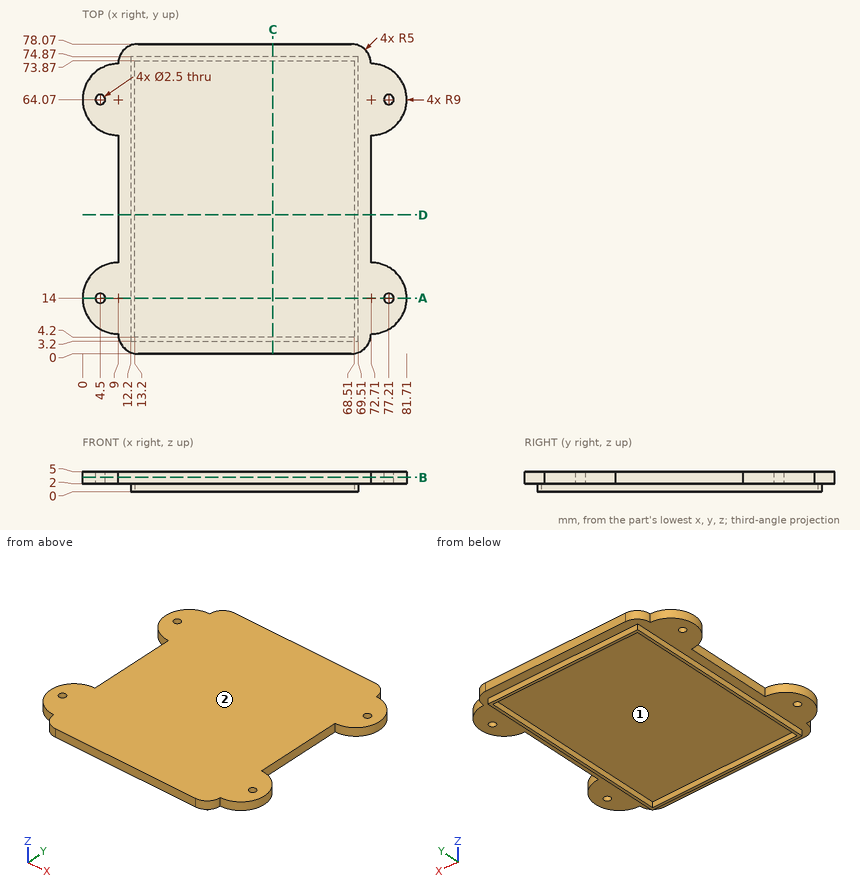
Could you check a few things on this drawing? It's one solid part, dimensions in mm from its lowest x, y, z. Give positions to 0.01 mm unless a question says otherwise; leave off trailing zeros. Order: outer loops, then holes, each group sorted by start corner. A loop starts at its lowest first (then second) coordinate and runs counter-clockwise, first axis right, second up. Notation, with made-up numbers: (34, 61.25) -> (66, 61.25) arc R34 ccw to (66, 94.25) -> close; hole circle Ø10 at (54.5, 6.25). An arc over 180 degrees is marked (long way). Answer in a Markdown table with one row per item. Add a question column.
Item 1: I'm going to push flat-ended pins straight in: P1, Ø2, axis at y = 49.5, z = 1.5, coming from the -X side; P2, Ø2.5, axis at y = 37, z = 3.5, coming from the +X side; P3, Ø1, axis at x = 54, z = 1, coming from the +Y side; P4, Ø1.5, axis at x = 77.21, y = 64.07, coming from the -Z side. Where does each tip first touch, or does it pass through?
Item 2: Please list where these lines run through material, in increasing order: probe 1 along X at (y, z) = (34, 1.85); probe 2 along Y at (x, z) = (54, 1.4); probe 3 along Y at (x, z) = (77.21, 4).
Item 3: Imagine slicing it at D-D (y = 35). List the corners of the cut face in (x, z) for me, and give its area (3 significant figures).
Item 4: Imagine slicing it at C-C (x = 48). List the corners of the cut face in (y, z) for me.
Item 5: Imagine slicing it at A-A (y = 14). List the corners of the cut face in (x, z) for me.
Item 6: We'd pull the mould along X, two halves only. Please class the marked faces 1 and 2: pulls with the +X half, pulls with the -X half, needs draft (parallel to the pull), parting line crosses it, or undercut.
Item 7: Imagine slicing it at B-B (z = 3.6). List the corners of the cut face in (x, y) for me.
Result:
| question | item | result |
|---|---|---|
| 1 | P1 | x = 9 |
| 1 | P2 | x = 72.71 |
| 1 | P3 | y = 74.87 |
| 1 | P4 | through |
| 2 | probe 1 | 12.2 to 13.2, 68.51 to 69.51 |
| 2 | probe 2 | 3.2 to 4.2, 73.87 to 74.87 |
| 2 | probe 3 | 6.21 to 12.75, 15.25 to 21.79, 56.28 to 62.82, 65.32 to 71.86 |
| 3 | outline | (9, 2) -> (12.2, 2) -> (12.2, 0) -> (13.2, 0) -> (13.2, 2) -> (68.51, 2) -> (68.51, 0) -> (69.51, 0) -> (69.51, 2) -> (72.71, 2) -> (72.71, 5) -> (9, 5) -> close |
| 3 | area | 195 mm2 |
| 4 | outline | (0, 2) -> (3.2, 2) -> (3.2, 0) -> (4.2, 0) -> (4.2, 2) -> (73.87, 2) -> (73.87, 0) -> (74.87, 0) -> (74.87, 2) -> (78.07, 2) -> (78.07, 5) -> (0, 5) -> close |
| 5 | outline | (0, 2) -> (3.25, 2) -> (3.25, 5) -> (0, 5) -> close; (5.75, 2) -> (12.2, 2) -> (12.2, 0) -> (13.2, 0) -> (13.2, 2) -> (68.51, 2) -> (68.51, 0) -> (69.51, 0) -> (69.51, 2) -> (75.96, 2) -> (75.96, 5) -> (5.75, 5) -> close; (78.46, 2) -> (81.71, 2) -> (81.71, 5) -> (78.46, 5) -> close |
| 6 | face 1 | undercut |
| 6 | face 2 | needs draft |
| 7 | outline | (9, 5) arc R5 ccw to (14, 0) -> (67.71, 0) arc R5 ccw to (72.71, 5) arc R9 ccw to (72.71, 23) -> (72.71, 55.07) arc R9 ccw to (72.71, 73.07) arc R5 ccw to (67.71, 78.07) -> (14, 78.07) arc R5 ccw to (9, 73.07) arc R9 ccw to (9, 55.07) -> (9, 23) arc R9 ccw to start; hole circle Ø2.5 at (4.5, 14); hole circle Ø2.5 at (4.5, 64.07); hole circle Ø2.5 at (77.21, 14); hole circle Ø2.5 at (77.21, 64.07) |
